```python
from build123d import *

# Parameters (mm, degrees)
SKETCH_1_R          = 17.35
SKETCH_1_R_2        = 5.5
EXTRUDE_1_DEPTH     = 3.5
SKETCH_6_R          = 1
CUT_EXTRUDE_3_DEPTH = 5
SKETCH_7_R          = 1.91
CUT_EXTRUDE_4_DEPTH = 2.08


with BuildPart() as part:
    # 草图1 → 凸台-拉伸1 (new body)
    with BuildSketch(Plane(origin=(0, 0, 0), x_dir=(1, 0, 0), z_dir=(0, 1, 0))):
        with Locations(Location((0, 0, 0), (0, 0, 270))):
            Circle(SKETCH_1_R)
        with Locations(Location((0, 0, 0), (0, 0, 270))):
            Circle(SKETCH_1_R_2, mode=Mode.SUBTRACT)
    extrude(amount=EXTRUDE_1_DEPTH)

    # 草图6 → 切除-拉伸3 (cut, symmetric)
    with BuildSketch(Plane(origin=(0, 0, 0), x_dir=(1, 0, 0), z_dir=(0, 1, 0))):
        with Locations(Location((8.131727984, 8.131727984, 0), (0, 0, 270))):
            Circle(SKETCH_6_R)
        with Locations(Location((7.424621202, -7.424621202, 0), (0, 0, 270))):
            Circle(SKETCH_6_R)
        with Locations(Location((-8.131727984, -8.131727984, 0), (0, 0, 270))):
            Circle(SKETCH_6_R)
        with Locations(Location((-7.424621202, 7.424621202, 0), (0, 0, 270))):
            Circle(SKETCH_6_R)
    extrude(amount=CUT_EXTRUDE_3_DEPTH, both=True, mode=Mode.SUBTRACT)

    # 草图7 → 切除-拉伸4 (cut)
    with BuildSketch(Plane(origin=(0, 3.5, 0), x_dir=(1, 0, 0), z_dir=(0, 1, 0))):
        with Locations(Location((-7.424621202, 7.424621202, 0), (0, 0, 270))):
            Circle(SKETCH_7_R)
        with Locations(Location((8.131727984, 8.131727984, 0), (0, 0, 270))):
            Circle(SKETCH_7_R)
        with Locations(Location((7.424621202, -7.424621202, 0), (0, 0, 270))):
            Circle(SKETCH_7_R)
        with Locations(Location((-8.131727984, -8.131727984, 0), (0, 0, 270))):
            Circle(SKETCH_7_R)
    extrude(amount=-CUT_EXTRUDE_4_DEPTH, mode=Mode.SUBTRACT)


solid = part.part
```
Work out the finished part from the listing and answer in its coordinate system (mm). A direction names the side the tool comes from. Round coordinates to 2 decimals unless told otherwise and drop trailing zeros. Loops run counter-clockwise (first coordinate to the right, second up) from the corner with the lowest first, then second, coordinate; pieces in that order, holes last.
(1) Find the intervals of material crossed by L1, parallel to X at y = 2.7, z = -7; L2, parallel to Z at x = 7, y = 2.7; L3, parallel to Z at x = 8, y = 2.9, in increasing order.
Computed values:
L1: x = -15.88 to -9.29, -5.56 to 6.59, 9.67 to 15.88
L2: z = -15.88 to -9.67, -6.59 to 5.56, 9.29 to 15.88
L3: z = -15.4 to -10.04, -6.23 to 5.6, 9.25 to 15.4
(2) The mould has two halves that part along X. Classify faces 3 (the cylindrical face through (5.21, 1.73, 16.55)), 4 (the flat face through (4, 3.5, -4)), 5 (the cylindrical face through (-5.53, 2.47, -7.67)): pulls with the +X half, pulls with the -X half, needs draft (parallel to the pull), parting line crosses it, or undercut.
Computed values:
face 3: parting line crosses it
face 4: needs draft
face 5: undercut
(3) Each of these flat-tipped pins is pushed along its axis until it touches: P1, Ø1.9, axis at x = 8.5, z = -8, coming from the +Y side; P2, Ø2, axis at y = 1, z = -2, coming from the -X side; P3, Ø1, axis at y = 1, z = 11.5, coming from the -X side. Where does it stop, or does it pass through?
Computed values:
P1: stops at y = 1.42
P2: stops at x = -17.32
P3: stops at x = -13.42
(4) The part is cut by section C-C, the plane y = 0.55. Give the vertices of the cut face in (x, z).
Computed values:
outline: circle Ø34.7 at (0, 0); hole circle Ø2 at (-8.13, 8.13); hole circle Ø2 at (-7.42, -7.42); hole circle Ø11 at (0, 0); hole circle Ø2 at (7.42, 7.42); hole circle Ø2 at (8.13, -8.13)
(5) For faces 1 (the flat face through (4, 0, -4)), 2 (the flat face through (-8.25, 1.42, -6.6)), determine the directions among +Z, -Z, +X, -X, +Y, -Y from which every point of the face is accessible in a straight line to the end or side of a thin tool.
Computed values:
face 1: +Z, -Z, +X, -X, -Y
face 2: +Y
(6) The part is cut by section D-D, the plane z = -13. Give the vertices of the cut face in (x, y).
Computed values:
outline: (-11.49, 0) - (11.49, 0) - (11.49, 3.5) - (-11.49, 3.5) - close
(7) The part is cut by section B-B, the plane x = 0. Give the vertices of the cut face in (y, z).
Computed values:
outline: (0, -17.35) - (3.5, -17.35) - (3.5, -5.5) - (0, -5.5) - close; (0, 5.5) - (3.5, 5.5) - (3.5, 17.35) - (0, 17.35) - close
(8) The part is cut by section A-A, the plane z = 0. Give the vertices of the cut face in (x, y), and give its area (4 significant figures).
Computed values:
outline: (-17.35, 0) - (-5.5, 0) - (-5.5, 3.5) - (-17.35, 3.5) - close; (5.5, 0) - (17.35, 0) - (17.35, 3.5) - (5.5, 3.5) - close
area: 82.95 mm2
